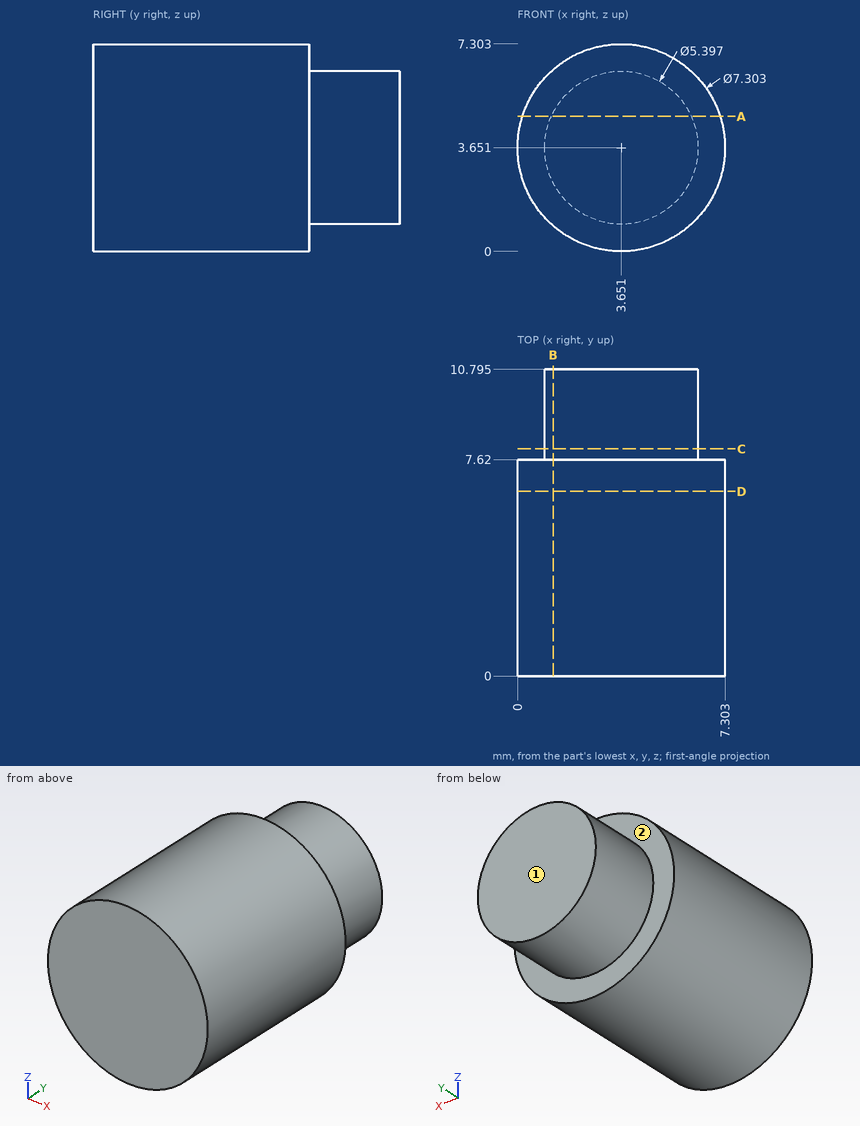
The figure shows three views and two pictorial views of one solid part (mm, origin at its lowest corner). Answer the questions. A direction names the side the tool comes from. Round coordinates to 2 decimals unless told otherwise and drop trailing zeros. Write each loop counter-clockwise with the first axis right and the second up, starting at its lowest first coordinate (ties: lowest second). Pieces come first, ordered by that corner, then holes. Notation, with made-up numbers: (61, -19) - (116, -19) arc R29 ccw to (116, 2) - close; hole circle Ø4 at (57, 21.5). An arc over 180 degrees is marked (long way). One line per question, with ' | ' between items. Start each with the question number.
1. Each of these flat-tipped pins is pushed along its axis until it touches: pin 1 (4 mm diameter, centred on y = 3, z = 1.5, fed in from +X); pin 2 (1 mm diameter, centred on x = 5.5, y = 2.5, fed in from +Z) (1 decimal). Where does it stop, or does it pass through?
2. Section C-C (y = 8) is taken. Determine the outline of the cut face in (x, z).
3. Section A-A (z = 4.75) is taken. Determine the outline of the cut face in (x, y) (1 decimal), and give its area (3 significant figures).
4. Section B-B (x = 1.25) is taken. Determine the outline of the cut face in (y, z) (1 decimal).
5. Section D-D (y = 6.5) is taken. Determine the outline of the cut face in (x, z).
6. Find the intervals of material crossed by probe 1 along Y at (x, z) = (0.5, 4.5); probe 2 along X at (y, z) = (2.5, 3.5); probe 3 along X at (y, z) = (6.75, 4.75), in increasing order. Write a range as [from, to].
7. For the marked faces 1 and 2, determine the directions among +Z, -Z, +X, -X, +Y, -Y from which every point of the face is accessible in a straight line to the end or side of a thin tool.
Filled in:
1) pin 1: x = 7.3 | pin 2: z = 7
2) outline: circle Ø5.4 at (3.65, 3.65)
3) outline: (0.2, 0) - (7.1, 0) - (7.1, 7.6) - (6.1, 7.6) - (6.1, 10.8) - (1.2, 10.8) - (1.2, 7.6) - (0.2, 7.6) - close | area: 68.7 mm²
4) outline: (0, 0.9) - (7.6, 0.9) - (7.6, 2.4) - (10.8, 2.4) - (10.8, 4.9) - (7.6, 4.9) - (7.6, 6.4) - (0, 6.4) - close
5) outline: circle Ø7.3 at (3.65, 3.65)
6) probe 1: [0, 7.62] | probe 2: [0, 7.3] | probe 3: [0.17, 7.13]
7) face 1: +Z, -Z, +X, -X, +Y | face 2: +Y
